```python
from build123d import *

# Parameters (mm, degrees)
SZKIC1_R                    = 3
DODANIE_WYCI_GNI_CIE1_DEPTH = 30
SZKIC2_W                    = 12
SZKIC2_H                    = 17
WYTNIJ_WYCI_GNI_CIE1_DEPTH  = 65.915329468
SZKIC3_R                    = 5
DODANIE_WYCI_GNI_CIE2_DEPTH = 30
ZAOKR_GLENIE3_R             = 2
ZAOKR_GLENIE6_RADIUS        = 8.5
ZAOKR_GLENIE6_LENGTH        = 9
ZAOKR_GLENIE7_RADIUS        = 8.5
ZAOKR_GLENIE7_LENGTH        = 9
ZAOKR_GLENIE8_RADIUS        = 8.5
ZAOKR_GLENIE8_LENGTH        = 9
ZAOKR_GLENIE9_RADIUS        = 8.5
ZAOKR_GLENIE9_LENGTH        = 9


with BuildPart() as part:
    # Szkic1 → Dodanie-wyci_gni_cie1 (new body)
    with BuildSketch(Plane.XY):
        Polygon((0, 0), (0, 17), (55, 17), (55, 0), (10, 0), align=None)
        with Locations((48, 9)):
            Circle(SZKIC1_R, mode=Mode.SUBTRACT)
        with Locations((7, 9)):
            Circle(SZKIC1_R, mode=Mode.SUBTRACT)
    extrude(amount=DODANIE_WYCI_GNI_CIE1_DEPTH)

    # Szkic2 → Wytnij-wyci_gni_cie1 (cut, through all)
    with BuildSketch(Plane(origin=(55, 0, 0), x_dir=(0, 0, -1), z_dir=(1, 0, 0))):
        with Locations((-15, 8.5)):
            Rectangle(SZKIC2_W, SZKIC2_H)
    extrude(amount=-WYTNIJ_WYCI_GNI_CIE1_DEPTH, mode=Mode.SUBTRACT)


with BuildPart() as wytnij_wyci_gni_cie1_piece_1:
    # of the separate pieces the step leaves, piece 1, a body of its own (wytnij_wyci_gni_cie1_pieces)
    add(part.part.solids().sort_by_distance((0, 0, 21))[0])



with BuildPart() as wytnij_wyci_gni_cie1_piece_2:
    # of the separate pieces the step leaves, piece 2, a body of its own (wytnij_wyci_gni_cie1_pieces)
    add(part.part.solids().sort_by_distance((0, 0, 0))[0])


with BuildPart() as wytnij_wyci_gni_cie1_piece_1_1:
    add(wytnij_wyci_gni_cie1_piece_1.part)

    add(wytnij_wyci_gni_cie1_piece_2.part)  # Dodanie-wyci_gni_cie2 merges Wytnij-wyci_gni_cie1 piece 2
    # Szkic3 → Dodanie-wyci_gni_cie2 (add)
    with BuildSketch(Plane(origin=(0, 0, 0), x_dir=(-1, 0, 0), z_dir=(0, 0, -1))):
        with Locations((-27.5, 8.5)):
            Circle(SZKIC3_R)
    extrude(amount=-DODANIE_WYCI_GNI_CIE2_DEPTH)

    # Zaokr_glenie3
    zaokr_glenie3_edges = [wytnij_wyci_gni_cie1_piece_1_1.edges().sort_by_distance(p)[0] for p in [
        (32.5, 8.5, 9),
        (32.5, 8.5, 21),
    ]]
    fillet(zaokr_glenie3_edges, radius=ZAOKR_GLENIE3_R)

    # Zaokr_glenie6: full round fillet: the end face becomes a half cylinder, R = half its width
    zaokr_glenie6_face = Plane((55, 8.5, 4.5), x_dir=(0, 0, 1), z_dir=(1, 0, 0))  # on the end face: x along it, z out of the body
    zaokr_glenie6_slab = zaokr_glenie6_face.offset(-ZAOKR_GLENIE6_RADIUS / 2) * Box(ZAOKR_GLENIE6_LENGTH, 2 * ZAOKR_GLENIE6_RADIUS, ZAOKR_GLENIE6_RADIUS, mode=Mode.PRIVATE)  # the body's end, R deep
    zaokr_glenie6_round = Plane((46.5, 8.5, 4.5), x_dir=(1, 0, 0), z_dir=(0, 0, 1)) * Cylinder(ZAOKR_GLENIE6_RADIUS, ZAOKR_GLENIE6_LENGTH, mode=Mode.PRIVATE)  # its axis R under the face
    add(zaokr_glenie6_slab - zaokr_glenie6_round, mode=Mode.SUBTRACT)

    # Zaokr_glenie7: full round fillet: the end face becomes a half cylinder, R = half its width
    zaokr_glenie7_face = Plane((55, 8.5, 25.5), x_dir=(0, 0, 1), z_dir=(1, 0, 0))  # on the end face: x along it, z out of the body
    zaokr_glenie7_slab = zaokr_glenie7_face.offset(-ZAOKR_GLENIE7_RADIUS / 2) * Box(ZAOKR_GLENIE7_LENGTH, 2 * ZAOKR_GLENIE7_RADIUS, ZAOKR_GLENIE7_RADIUS, mode=Mode.PRIVATE)  # the body's end, R deep
    zaokr_glenie7_round = Plane((46.5, 8.5, 25.5), x_dir=(1, 0, 0), z_dir=(0, 0, 1)) * Cylinder(ZAOKR_GLENIE7_RADIUS, ZAOKR_GLENIE7_LENGTH, mode=Mode.PRIVATE)  # its axis R under the face
    add(zaokr_glenie7_slab - zaokr_glenie7_round, mode=Mode.SUBTRACT)

    # Zaokr_glenie8: full round fillet: the end face becomes a half cylinder, R = half its width
    zaokr_glenie8_face = Plane((0, 8.5, 4.5), x_dir=(0, 0, 1), z_dir=(-1, 0, 0))  # on the end face: x along it, z out of the body
    zaokr_glenie8_slab = zaokr_glenie8_face.offset(-ZAOKR_GLENIE8_RADIUS / 2) * Box(ZAOKR_GLENIE8_LENGTH, 2 * ZAOKR_GLENIE8_RADIUS, ZAOKR_GLENIE8_RADIUS, mode=Mode.PRIVATE)  # the body's end, R deep
    zaokr_glenie8_round = Plane((8.5, 8.5, 4.5), x_dir=(-1, 0, 0), z_dir=(0, 0, 1)) * Cylinder(ZAOKR_GLENIE8_RADIUS, ZAOKR_GLENIE8_LENGTH, mode=Mode.PRIVATE)  # its axis R under the face
    add(zaokr_glenie8_slab - zaokr_glenie8_round, mode=Mode.SUBTRACT)

    # Zaokr_glenie9: full round fillet: the end face becomes a half cylinder, R = half its width
    zaokr_glenie9_face = Plane((0, 8.5, 25.5), x_dir=(0, 0, -1), z_dir=(-1, 0, 0))  # on the end face: x along it, z out of the body
    zaokr_glenie9_slab = zaokr_glenie9_face.offset(-ZAOKR_GLENIE9_RADIUS / 2) * Box(ZAOKR_GLENIE9_LENGTH, 2 * ZAOKR_GLENIE9_RADIUS, ZAOKR_GLENIE9_RADIUS, mode=Mode.PRIVATE)  # the body's end, R deep
    zaokr_glenie9_round = Plane((8.5, 8.5, 25.5), x_dir=(-1, 0, 0), z_dir=(0, 0, -1)) * Cylinder(ZAOKR_GLENIE9_RADIUS, ZAOKR_GLENIE9_LENGTH, mode=Mode.PRIVATE)  # its axis R under the face
    add(zaokr_glenie9_slab - zaokr_glenie9_round, mode=Mode.SUBTRACT)


solid = wytnij_wyci_gni_cie1_piece_1_1.part
```
CAD build for the part. Positions are in the model's coordinates, mm. A direction names the side the tool comes from. Round coordinates to 2 decimals unless told otherwise and drop trailing zeros. Order: outer loops, then holes, each group sorted by start corner. A loop starts at its lowest first (then second) coordinate and runs counter-clockwise, first axis right, second up. Notation, with made-up numbers: (-30.75, 85) - (20.25, 85) arc R16 ccw to (20.25, 93) - close; hole circle Ø1 at (75, 9.5). An arc over 180 degrees is marked (long way). Answer as CSV lines item,"result". Start each with the question number.
1. Saw through at C-C, the plane x = 14. Write the cut outline in (y, z), and give its area (3 significant figures).
2. Saw through at D-D, the plane x = 48. Write the cut outline in (y, z), and give its area (3 significant figures).
3. Tool access for faces 1 (the face through (0.002, 8.687, 4.563)), 2 (the face through (31.185, 11.879, 14.944)): list every direction of +Z, -Z, +X, -X, +Y, -Y with a clear straight run to the whole face (end or side of a thin tool).
4. Saw through at A-A, the plane x = 27.5. Write the cut outline in (y, z), and give its area (3 significant figures).
5. Pull direction X, two halves, no side cores. Call faces 3 (the face through (9.77, 7.85, 4.44)), 4 (the face through (54.998, 8.313, 25.563)), 5 (the face through (27, 17, 25)): +X half, -X half, draft (parallel to the pull), parting line (faces both ways), or undercut.
6. Drill centre lines: L1, parallel to Z at x = 11, y = 7.75; L2, parallel to X at y = 9, z = 24.5; L3, parallel to X at y = 9.5, z = 4.5. Where is each one in solid material? Low to high. Write a range as [from, to].
7. Saw through at B-B, the plane z = 22.5. Write the cut outline in (x, y), and give its area (3 significant figures).
8. Pin check, flat tips, straight feed: pin 1 (8.5 mm diameter, centred on x = 20.5, y = 8.5, fed in from -Z); pin 2 (1.5 mm diameter, centred on y = 5.5, z = 22.5, fed in from -X); pin 3 (5 mm diameter, centred on y = 6.5, z = 18, fed in from +X); pin 4 (5 mm diameter, centred on x = 32.5, z = 15.5, fed in from -Y). Stop position of each tip, or through.
Model answer:
1,outline,"(0, 0) - (17, 0) - (17, 9) - (0, 9) - close; (0, 21) - (17, 21) - (17, 30) - (0, 30) - close"
1,area,"306 mm²"
2,outline,"(0.13, 0) - (6, 0) - (6, 9) - (0.13, 9) - close; (0.13, 21) - (6, 21) - (6, 30) - (0.13, 30) - close; (12, 0) - (16.87, 0) - (16.87, 9) - (12, 9) - close; (12, 21) - (16.87, 21) - (16.87, 30) - (12, 30) - close"
2,area,"193 mm²"
3,face 1,"+Z, -Z, -X"
3,face 2,"none"
4,outline,"(0, 0) - (17, 0) - (17, 9) - (15.5, 9) arc R2 cw to (13.5, 11) - (13.5, 19) arc R2 cw to (15.5, 21) - (17, 21) - (17, 30) - (0, 30) - (0, 21) - (1.5, 21) arc R2 cw to (3.5, 19) - (3.5, 11) arc R2 cw to (1.5, 9) - (0, 9) - close"
4,area,"429 mm²"
5,face 3,"undercut"
5,face 4,"+X half"
5,face 5,"draft"
6,L1,"z = [0, 9], [21, 30]"
6,L2,"x = [0.01, 4], [10, 45], [51, 54.99]"
6,L3,"x = [0.06, 4.04], [9.96, 45.04], [50.96, 54.94]"
7,outline,"(8.5, 0) - (46.5, 0) arc R8.5 ccw to (46.5, 17) - (8.5, 17) arc R8.5 ccw to start; hole circle Ø6 at (7, 9); hole circle Ø6 at (48, 9)"
7,area,"816 mm²"
8,pin 1,"stops at z = 0"
8,pin 2,"stops at x = 0.3"
8,pin 3,"stops at x = 32.92"
8,pin 4,"stops at y = 4.17"
